from build123d import *

# Parameters (mm, degrees)
BOSS_EXTRUDE1_DEPTH      = 457.2
BOSS_EXTRUDE1_DEPTH_BACK = 38.1
SKETCH1_W                = 19.558
SKETCH1_H                = 19.558
SKETCH2_R                = 3.6195
CUT_EXTRUDE1_DEPTH       = 38.1
SKETCH3_W                = 127
SKETCH3_H                = 19.558
BOSS_EXTRUDE2_DEPTH      = 19.05


with BuildPart() as part:
    # Sketch1 → Boss-Extrude1 (new, two sides: drawn at the far end of the back side and taken through both)
    with BuildSketch(Plane.ZY.offset(17.272).offset(-BOSS_EXTRUDE1_DEPTH_BACK)):
        with Locations((44.45, 101.6)):
            Rectangle(SKETCH1_W, SKETCH1_H)
    extrude(amount=BOSS_EXTRUDE1_DEPTH + BOSS_EXTRUDE1_DEPTH_BACK)

    # Sketch2 → Cut-Extrude1 (cut)
    with BuildSketch(Plane(origin=(20.828, 0, 0), x_dir=(0, 0, -1), z_dir=(1, 0, 0))):
        with Locations((-44.45, 101.6)):
            Circle(SKETCH2_R)
    extrude(amount=-CUT_EXTRUDE1_DEPTH, mode=Mode.SUBTRACT)

    # Sketch3 → Boss-Extrude2 (add)
    with BuildSketch(Plane.XY.offset(54.229)):
        with Locations((-42.672, 101.6)):
            Rectangle(SKETCH3_W, SKETCH3_H)
    extrude(amount=BOSS_EXTRUDE2_DEPTH)


solid = part.part
Could you check a few things on this model? Use its own coordinates, in mm. A direction names the side the tool comes from. Coordinates: 2 decimals unless noted, no trailing zeros. Write each loop counter-clockwise with the first axis right and the second up, starting at its lowest first coordinate (ties: lowest second). Pieces come first, ordered by that corner, then holes. Notation, with made-up numbers: (47.5, 53) - (100.5, 53) arc R8 ccw to (100.5, 67) - close; hole circle Ø6 at (82.25, 54). An arc over 180 degrees is marked (long way). Write item = value, one per line.
1) Please list where these lines run through material, in increasing order: line 1 (Y direction, x = 12, z = 44); line 2 (Z direction, x = -147, y = 109.5); line 3 (X direction, y = 101.5, z = 68.5). Write a range as [from, to].
Result set:
line_1 = [91.82, 98.01], [105.19, 111.38]
line_2 = [34.67, 54.23]
line_3 = [-106.17, 20.83]
2) Suppose I cut it at A-A on y = 101.6. Please give me the cut outline in (x, z), plus the area to 3 significant figures.
Result set:
outline = (-474.47, 34.67) - (20.83, 34.67) - (20.83, 40.83) - (-17.27, 40.83) - (-17.27, 48.07) - (20.83, 48.07) - (20.83, 73.28) - (-106.17, 73.28) - (-106.17, 54.23) - (-474.47, 54.23) - close
area = 11,800 mm2
3) For faces 1 (the flat face through (-175, 111.379, 49)), 2 (the flat face through (-106.172, 101, 64)), which set-ups out of +Z, -Z, +X, -X, +Y, -Y let a thin tool reach every point of the face, with its end or its side?
Result set:
face_1 = +Z, -Z, +X, -X, +Y
face_2 = +Z, -X, +Y, -Y
4) Will these pins go through, and if not, where does the flat tip stop? pin 1 Ø1.5 at (x, y) = (-321.5, 109) entering from +Z; pin 2 Ø3.5 at (y, z) = (102, 46) entering from +X.
Result set:
pin_1 = 54.23
pin_2 = -17.27
5) Suppose I cut it at B-B on x = -350. Please give me the cut outline in (y, z).
Result set:
outline = (91.82, 34.67) - (111.38, 34.67) - (111.38, 54.23) - (91.82, 54.23) - close
6) Suppose I cut it at C-C on z = 61. Please give me the cut outline in (x, y).
Result set:
outline = (-106.17, 91.82) - (20.83, 91.82) - (20.83, 111.38) - (-106.17, 111.38) - close
